Design review of the part built by this model. Coordinates are the model's own, in mm. A direction names the side the tool comes from. Give positions to 0.01 mm unless a question says otherwise; leave off trailing zeros. Loops run counter-clockwise (first coordinate to the right, second up) from the corner with the lowest first, then second, coordinate; pieces in that order, holes last. Notation, with made-up numbers: (50, 70) -> (103, 70) arc R19 ccw to (103, 90) -> close; hole circle Ø5 at (85.5, 39). An arc over 180 degrees is marked (long way). Answer in a Markdown table with one row per item. Add a question column.
(1) For faces 1 (the flat face through (40, 215, 25)), 2 (the flat face through (60, 215, 25)), 3 (the flat face through (50, 215, 35)), 4 (the flat face through (50, 215, 15)), list the 3-axis set-ups (+Z, -Z, +X, -X, +Y, -Y) from which the entire face can be reached by the end or side of a thin tool; tool diameter is ignored.
(2) For line 1 (X direction, y = 15.5, z = 25.5); line 2 (Z direction, x = 41.5, y = 214); line 3 (X direction, y = 68.5, z = 12.5), list the stretches that pass through material, from the lowest coordinate up.
(3) Consider section D-D on z = 41. Write out the cut boundary in (x, y).
(4) For pin 1 (6 mm diameter, centred on y = 222.5, z = 27, fed in from -X); pin 2 (3 mm diameter, centred on x = 25, z = 23.5, fed in from +Y); pin 3 (22 mm diameter, centred on x = 47.5, y = 212.5, fed in from -Z), all flat-tipped, find the tip position at first contact; note any pin that passes through.
(5) Consider section A-A on z = 23.5. Write out the cut boundary in (x, y), then the cut area to 3 significant figures.
(6) Consider section B-B on x = 43. Write out the cut boundary in (y, z) (3 decimals).
(7) Consider section C-C on y = 98.5. Write out the cut boundary in (x, z), then the cut area to 3 significant figures.
from build123d import *

# Parameters (mm, degrees)
SALIENTE_EXTRUIR3_DEPTH = 50
CROQUIS3_W              = 20
CROQUIS3_H              = 20
SALIENTE_EXTRUIR4_DEPTH = 30


with BuildPart() as part:
    # Croquis2 → Saliente-Extruir3 (new body)
    with BuildSketch(Plane.XY):
        Polygon((0, 200), (0, 110), (80, 0), (90, 0), (90, 200), align=None)
    extrude(amount=SALIENTE_EXTRUIR3_DEPTH)

    # Croquis3 → Saliente-Extruir4 (add)
    with BuildSketch(Plane(origin=(0, 200, 0), x_dir=(1, 0, 0), z_dir=(0, 1, 0))):
        with Locations((50, -25)):
            Rectangle(CROQUIS3_W, CROQUIS3_H)
    extrude(amount=SALIENTE_EXTRUIR4_DEPTH)


solid = part.part
Values follow:
| question | item | result |
|---|---|---|
| 1 | face 1 | +Z, -Z, -X, +Y |
| 1 | face 2 | +Z, -Z, +X, +Y |
| 1 | face 3 | +Z, +X, -X, +Y |
| 1 | face 4 | -Z, +X, -X, +Y |
| 2 | line 1 | 68.73 to 90 |
| 2 | line 2 | 15 to 35 |
| 2 | line 3 | 30.18 to 90 |
| 3 | outline | (0, 110) -> (80, 0) -> (90, 0) -> (90, 200) -> (0, 200) -> close |
| 4 | pin 1 | x = 40 |
| 4 | pin 2 | y = 200 |
| 4 | pin 3 | z = 15 |
| 5 | outline | (0, 110) -> (80, 0) -> (90, 0) -> (90, 200) -> (60, 200) -> (60, 230) -> (40, 230) -> (40, 200) -> (0, 200) -> close |
| 5 | area | 14,200 mm2 |
| 6 | outline | (50.875, 0) -> (200, 0) -> (200, 15) -> (230, 15) -> (230, 35) -> (200, 35) -> (200, 50) -> (50.875, 50) -> close |
| 7 | outline | (8.36, 0) -> (90, 0) -> (90, 50) -> (8.36, 50) -> close |
| 7 | area | 4,080 mm2 |
